Work out the finished part from the listing and answer in its coordinate system (mm). A direction names the side the tool comes from. Give positions to 0.01 mm unless a question says otherwise; leave off trailing zeros. Loops run counter-clockwise (first coordinate to the right, second up) from the corner with the lowest first, then second, coordinate; pieces in that order, holes last. Notation, with made-up numbers: M -17,45 L 19,45 A25 ccw 19,84 Z; hole C 71,48 d2. An arc over 180 degrees is marked long. Answer in a Markdown table with one row per item. Add a question column.
Autodesk Inventor part; units mm, degrees
ref_plane "YZ Plane" through (0, 0, 0) normal (1, 0, 0) x (0, 1, 0)
ref_plane "XZ Plane" through (0, 0, 0) normal (0, 1, 0) x (-1, 0, 0)
ref_plane "XY Plane" through (0, 0, 0) normal (0, 0, 1) x (1, 0, 0)
sketch "Sketch1" plane through (0, 0, 0) normal (0, 1, 0) x (-1, 0, 0)
  point P0 (0, 0)
sketch "Sketch2" plane through (0, 0, 0) normal (0, 1, 0) x (-1, 0, 0)
  point P0 (0, 0)
sketch "Sketch3" plane through (0, 0, 0) normal (0, 1, 0) x (-1, 0, 0)
  line L0 (0, 0) -> (0, -8.75) construction
  line L1 (0, 0) -> (0, 8.75) construction
  line L2 (8.75, 8.75) -> (-8.75, 8.75)
  line L3 (-8.75, 8.75) -> (-8.75, -8.75)
  line L4 (-8.75, -8.75) -> (8.75, -8.75)
  line L5 (8.75, -8.75) -> (8.75, 8.75)
  circle A0 centre (8.75, 0) radius 8.75
  circle A1 centre (8.75, 0) radius 4.05
  line L6 (0, 0) -> (4.05, 0) construction
  dimension "d0" = 8.75
  dimension "d1" = 8.75
  dimension "d2" = 17.5
  dimension "d3" = 17.5
  dimension "d7" = 8.1
  dimension "d9" = 4.05
sketch "Sketch4" plane through (0, 0, 0) normal (0, 1, 0) x (-1, 0, 0)
  point P0 (0, 0)
sketch "Sketch5" plane through (0, 0, 0) normal (0, 1, 0) x (-1, 0, 0)
  point P0 (0, 0)
extrude "Extrusion2" add sketch "Sketch3" against normal blind 16 contours A0 L4 L3 L2 | A0 L5 A1 | L5 A1 A0 | L5 A1 picked at (7.639, -0.7669)
sketch "Sketch6" plane through (0, 0, 0) normal (0, 1, 0) x (1, 0, 0)
  line L0 (-8.75, 4.05) -> (-8.75, -4.05)
  circle A0 centre (-8.75, 0) radius 4.05
  point P0 (0, 0)
sketch "Sketch7" plane through (0, 0, 0) normal (0, 1, 0) x (1, 0, 0)
  line L0 (-8.75, 4.05) -> (-8.75, -4.05) construction
  circle A0 centre (-8.75, 0) radius 4.05 construction
  arc A1 (-8.75, 4.05) -> (-8.75, -4.05) centre (-8.75, 0) ccw construction
  arc A2 (-8.75, 8.75) -> (-8.75, -8.75) centre (-8.75, 0) ccw construction
  point P0 (0, 0)
  dimension "d12" = 8.1
extrude "Extrusion3" cut sketch "Sketch6" against normal blind 16
sketch "Sketch8" plane through (-8.75, 0, 8.75) normal (0, 0, 1) x (1, 0, 0)
  line L0 (17.5, -16) -> (0, -16) construction
  line L1 (8.75, -16) -> (8.75, 0) construction
  circle A0 centre (8.75, -8) radius 4.05
  dimension "d15" = 8.1
extrude "Extrusion4" cut sketch "Sketch8" against normal up to next
sketch "Sketch9" plane through (0, 0, 0) normal (0, 1, 0) x (1, 0, 0)
  point P0 (0, 0)
sketch "Sketch10" plane through (0, 0, 0) normal (0, 1, 0) x (1, 0, 0)
  point P0 (0, 0)
sketch "Sketch11" plane through (0, 0, 0) normal (0, 1, 0) x (1, 0, 0)
  point P0 (0, 0)
sketch "Sketch12" plane through (0, 0, 0) normal (0, 1, 0) x (1, 0, 0)
  line L0 (8.75, 8.75) -> (8.75, -8.75) construction
  line L1 (8.75, 8.75) -> (8.75, 2.5) construction
  line L2 (8.75, 2.5) -> (8.75, -2.5) construction
  line L3 (8.75, -2.5) -> (8.75, -8.75) construction
  circle A0 centre (-8.75, 0) radius 4.05
  line L4 (8.75, -2.5) -> (-5.5637, -2.5)
  line L5 (-5.5637, -2.5) -> (-5.5637, 2.5)
  line L6 (-5.5637, 2.5) -> (8.75, 2.5)
  line L7 (8.75, 2.5) -> (8.75, -2.5)
  point P0 (0, 0)
  dimension "d18" = 6.25
  dimension "d19" = 5
  dimension "d20" = 6.25
extrude "Extrusion5" cut sketch "Sketch12" against normal up to next contours A0 L5 | A0 L6 L7 L4 picked at (-5.4064, -0.5793)
properties part number "base and bar clamp"
(1) Section C-C, the plane x = 0 is taken. Determine the outline of the cut face in (y, z), and give its area (4 significant figures).
(2) Which of the six approach directions +Z, -Z, +X, -X, +Y, -Y give full straight-line access (tool end or side, diameter ignored) to faces 5 (the face through (8.75, -8, 6)), 6 (the face through (5, -8, 2.5))?
(3) The mould has two halves that part along X. Classify faces 1 (the face through (5, -8, -2.5)), 2 (the face through (-17.498, -7.888, -0.192)), 3 (the face through (8.75, -8, -6)), 4 (the face through (-0.878, -11.954, -5.581)): pulls with the +X half, pulls with the -X half, needs draft (parallel to the pull), parting line crosses it, or undercut.
(4) Consider line 1 along Z through (x, y) = (-4, -5.75); line 2 along Y through (x, z) = (0, -7.5); line 3 along Y through (x, z) = (-3.25, -4). Determine where each line is inside the solid, lowest interval first. Write a range as from..to.
(5) This flat-tipped pin is pushed along its axis until it touches: P1, Ø5, axis at x = -13, y = -5, coming from the +Z side. Where does it stop, or does it pass through?
(6) Section D-D, the plane x = -2.75 is taken. Determine the outline of the cut face in (y, z).
(7) Section B-B, the plane x = 6 is taken. Determine the outline of the cut face in (y, z), and give its area (3 significant figures).
Numbers:
| question | item | result |
|---|---|---|
| 1 | outline | M -16,-8.75 L -12.05,-8.75 L -12.05,-2.5 L -16,-2.5 Z; M -16,2.5 L -12.05,2.5 L -12.05,8.75 L -16,8.75 Z; M -3.95,-8.75 L 0,-8.75 L 0,-2.5 L -3.95,-2.5 Z; M -3.95,2.5 L 0,2.5 L 0,8.75 L -3.95,8.75 Z |
| 1 | area | 98.75 mm² |
| 2 | face 5 | +Z, -Z, +X, +Y, -Y |
| 2 | face 6 | +X, +Y, -Y |
| 3 | face 1 | needs draft |
| 3 | face 2 | pulls with the -X half |
| 3 | face 3 | pulls with the +X half |
| 3 | face 4 | undercut |
| 4 | line 1 | z = -8.75..-2.5, 2.5..8.75 |
| 4 | line 2 | y = -16..-12.05, -3.95..0 |
| 4 | line 3 | y = -16..-10.42, -5.58..0 |
| 5 | P1 | stops at z = 8.57 |
| 6 | outline | M -16,-8.75 L -10.97,-8.75 L -10.97,-2.5 L -16,-2.5 Z; M -16,2.5 L -10.97,2.5 L -10.97,8.75 L -16,8.75 Z; M -5.03,-8.75 L 0,-8.75 L 0,-2.5 L -5.03,-2.5 Z; M -5.03,2.5 L 0,2.5 L 0,8.75 L -5.03,8.75 Z |
| 7 | outline | M -16,-8.75 L 0,-8.75 L 0,-2.5 L -16,-2.5 Z; M -16,2.5 L 0,2.5 L 0,8.75 L -16,8.75 Z |
| 7 | area | 200 mm² |
